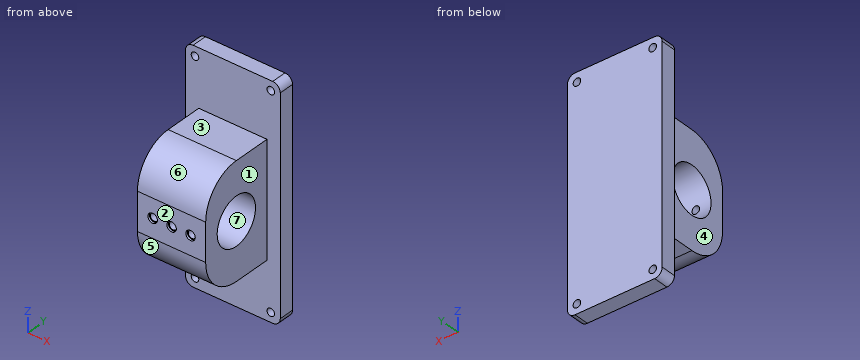
from build123d import *

# Parameters (mm, degrees)
SKETCH1_W                 = 50
SKETCH1_H                 = 120
BOSS_EXTRUDE1_DEPTH       = 8
SKETCH2_R                 = 2
CUT_EXTRUDE1_DEPTH        = 10
LPATTERN1_COUNT           = 2
LPATTERN1_PITCH           = 40
LPATTERN2_COUNT           = 2
LPATTERN2_PITCH           = 110
LPATTERN2_COPY_1_SKETCH_R = 2
LPATTERN2_COPY_1_DEPTH    = 10
BOSS_EXTRUDE2_DEPTH       = 40
SKETCH6_R                 = 12.5
CUT_EXTRUDE2_DEPTH        = 84.958322994
CUT_EXTRUDE3_DEPTH        = 84.958322994
FILLET1_R                 = 4
SKETCH8_R                 = 2
CUT_EXTRUDE4_DEPTH        = 10
SKETCH9_R                 = 2.5
CUT_EXTRUDE5_DEPTH        = 1
LPATTERN3_COUNT           = 2
LPATTERN3_PITCH           = 10
LPATTERN3_COL_COUNT       = 2
LPATTERN3_COL_PITCH       = 10


with BuildPart() as part:
    # Sketch1 → Boss-Extrude1 (new body)
    with BuildSketch(Plane(origin=(0, 0, 0), x_dir=(1, 0, 0), z_dir=(0, 1, 0))):
        with Locations((-110, 0)):
            Rectangle(SKETCH1_W, SKETCH1_H)
    extrude(amount=BOSS_EXTRUDE1_DEPTH)

    # Sketch2 → Cut-Extrude1 (cut)
    with BuildSketch(Plane(origin=(0, 8, 0), x_dir=(1, 0, 0), z_dir=(0, 1, 0))):
        with Locations(Location((-130, 55, 0), (0, 0, 270))):
            Circle(SKETCH2_R)
    cut_extrude1 = extrude(amount=-CUT_EXTRUDE1_DEPTH, mode=Mode.SUBTRACT)

    # LPattern1: Cut-Extrude1 ×2
    with Locations(*[(i * LPATTERN1_PITCH, 0, 0) for i in range(1, LPATTERN1_COUNT)]):
        add(cut_extrude1, mode=Mode.SUBTRACT)

    # LPattern2: Cut-Extrude1 ×2
    with Locations(*[(0, 0, i * LPATTERN2_PITCH) for i in range(1, LPATTERN2_COUNT)]):
        add(cut_extrude1, mode=Mode.SUBTRACT)

    # LPattern2 copy 1 sketch → LPattern2 copy 1 (cut)
    with BuildSketch(Plane(origin=(40, 8, 110), x_dir=(1, 0, 0), z_dir=(0, 1, 0))):
        with Locations(Location((-130, 55, 0), (0, 0, 270))):
            Circle(LPATTERN2_COPY_1_SKETCH_R)
    extrude(amount=-LPATTERN2_COPY_1_DEPTH, mode=Mode.SUBTRACT)

    # Sketch5 → Boss-Extrude2 (add)
    with BuildSketch(Plane.XZ):
        with BuildLine():
            Line((-92, 30), (-92, -30))
            ThreePointArc((-92, -30), (-110, -48), (-128, -30))
            Line((-128, -30), (-128, 30))
            ThreePointArc((-128, 30), (-110, 48), (-92, 30))
        make_face()
    extrude(amount=BOSS_EXTRUDE2_DEPTH)

    # Sketch6 → Cut-Extrude2 (cut, through all)
    with BuildSketch(Plane.ZY.offset(128)):
        with Locations((0, -20)):
            Circle(SKETCH6_R)
    extrude(amount=-CUT_EXTRUDE2_DEPTH, mode=Mode.SUBTRACT)

    # Sketch7 → Cut-Extrude3 (cut, through all)
    with BuildSketch(Plane(origin=(-92, 0, 0), x_dir=(0, 0, -1), z_dir=(1, 0, 0))):
        Polygon((-30, -20), (-30, 0), (-48, 0), (-48, -40), (-30, -40), align=None)
        with BuildLine():
            ThreePointArc((-10, -40), (-24.142135624, -34.142135624), (-30, -20))
            Line((-30, -20), (-30, -40))
            Line((-30, -40), (-10, -40))
        make_face()
        with BuildLine():
            ThreePointArc((30, -20), (24.142135624, -34.142135624), (10, -40))
            Line((10, -40), (30, -40))
            Line((30, -40), (30, -20))
        make_face()
        Polygon((30, -20), (30, -40), (48, -40), (48, 0), (30, 0), align=None)
    extrude(amount=-CUT_EXTRUDE3_DEPTH, mode=Mode.SUBTRACT)

    # Fillet1
    fillet1_edges = [part.edges().sort_by_distance(p)[0] for p in [
        (-85, 4, 60),
        (-135, 4, 60),
        (-135, 4, -60),
        (-85, 4, -60),
    ]]
    fillet(fillet1_edges, radius=FILLET1_R)

    # Sketch8 → Cut-Extrude4 (cut)
    with BuildSketch(Plane.XZ.offset(40)):
        with Locations(Location((-110, 0, 0), (0, 0, 270))):
            Circle(SKETCH8_R)
    cut_extrude4 = extrude(amount=-CUT_EXTRUDE4_DEPTH, mode=Mode.SUBTRACT)

    # Sketch9 → Cut-Extrude5 (cut)
    with BuildSketch(Plane.XZ.offset(40)):
        with Locations(Location((-110, 0, 0), (0, 0, 270))):
            Circle(SKETCH9_R)
    cut_extrude5 = extrude(amount=-CUT_EXTRUDE5_DEPTH, mode=Mode.SUBTRACT)

    # LPattern3: Cut-Extrude4, Cut-Extrude5 ×2
    with Locations(*[(i * LPATTERN3_PITCH, 0, 0) for i in range(1, LPATTERN3_COUNT)]):
        add(cut_extrude4, mode=Mode.SUBTRACT)
        add(cut_extrude5, mode=Mode.SUBTRACT)

    # LPattern3 col: Cut-Extrude4, Cut-Extrude5 ×2
    with Locations(*[(-i * LPATTERN3_COL_PITCH, 0, 0) for i in range(1, LPATTERN3_COL_COUNT)]):
        add(cut_extrude4, mode=Mode.SUBTRACT)
        add(cut_extrude5, mode=Mode.SUBTRACT)


solid = part.part
Model file for the job. Use its own axes, mm. Face numbers are marked on the shaded views. A direction names the side the tool comes from. Give positions to 0.01 mm unless a question says otherwise; leave off trailing zeros. Order: outer loops, then holes, each group sorted by start corner. A loop starts at its lowest first (then second) coordinate and runs counter-clockwise, first axis right, second up. Notation, with made-up numbers: (54.25, -8) - (84.25, -8) arc R18 cw to (84.25, 24) - close; hole circle Ø4 at (-38.5, 18). An arc over 180 degrees is marked (long way). Return JSON: item names as keys, results as strings.
1) Probe line 1 (X direction, y = 6.5, z = -55); line 2 (Y direction, x = -117, z = 0); line 3 (X direction, y = -34.75, z = 0). List the from-to ranges inside material, lowest first. Write a range as from..to.
Geometry says:
{"line 1": "-135..-132, -128..-92, -88..-85", "line 2": "-40..-32.5, -7.5..8", "line 3": "-128..-122, -118..-112, -108..-102, -98..-92"}
2) Cut at A-A, the plane y = -13.5. Give the cut face in (x, z).
Geometry says:
{"outline": "(-128, -30) - (-92, -30) - (-92, -10.68) - (-128, -10.68) - close; (-128, 10.68) - (-92, 10.68) - (-92, 30) - (-128, 30) - close"}
3) Cut at B-B, the plane z = 0. Count the separate pieces of the cut face and the enclosed holes in it, plus the area to 3 significant figures.
Geometry says:
{"separate pieces": "5", "enclosed holes": "0", "area": "847 mm²"}
4) Cut at D-D, the plane y = -3.5. Give the cut face in (x, z), plus the area to 3 significant figures.
Geometry says:
{"outline": "(-128, -30) - (-92, -30) - (-92, 30) - (-128, 30) - close", "area": "2,160 mm²"}
5) Cut at C-C, the plane x = -120. Give the cut face in (y, z).
Geometry says:
{"outline": "(-40, -10) arc R20 ccw to (-20, -30) - (0, -30) - (0, -60) - (8, -60) - (8, 60) - (0, 60) - (0, 30) - (-20, 30) arc R20 ccw to (-40, 10) - (-40, 2.5) - (-39, 2.5) - (-39, 2) - (-32.34, 2) arc R12.5 cw (long way) to (-32.34, -2) - (-39, -2) - (-39, -2.5) - (-40, -2.5) - close"}
6) 3-axis set-ups, long thin cutter, end or side, ignore diameter. For the marked faces 1, 2 and 3: which of +Z, -Z, +X, -X, +Y, -Y reach the whole face in a straight line?
Geometry says:
{"face 1": "+Z, -Z, +X, -Y", "face 2": "+Z, -Z, +X, -X, -Y", "face 3": "+Z, +X, -X, -Y"}
7) Flat gauge pins, fed straight in: P1, Ø1, axis at x = -107, y = -8, coming from the +Z side; P2, Ø10, axis at x = -127, z = -16, coming from the -Y side (3 decimals); P3, Ø6.5, axis at x = -90, z = -55, coming from the -Y side. Where does each tip first touch, or does it go through?
Geometry says:
{"P1": "z = 30", "P2": "y = -39.975", "P3": "y = 0"}
8) Pull direction Z, two halves, no side cores. Call the marked faces 4, 5, 6 and 7: pulls with the +Z half, pulls with the -Z half, needs draft (parallel to the pull), parting line crosses it, or undercut.
Geometry says:
{"face 4": "needs draft", "face 5": "pulls with the -Z half", "face 6": "pulls with the +Z half", "face 7": "undercut"}
